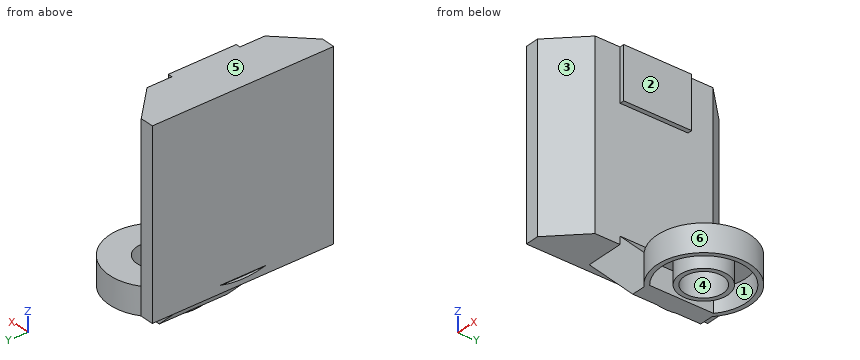
from build123d import *

# Parameters (mm, degrees)
F0_R     = 10.25
F0_R_2   = 4.25
F1_DEPTH = 6
F2_T     = -1
F4_DEPTH = 7.5
F6_DEPTH = 10
F7_SIZE  = 7


# Not quite as in the source:
# - a feature names something its author has since deleted; it is built from what else it names


with BuildPart() as f1:
    # F0 (on Top) → F1 (new body)
    with BuildSketch(Plane.XY):
        Circle(F0_R)
        Circle(F0_R_2, mode=Mode.SUBTRACT)
    extrude(amount=F1_DEPTH)

    # F2
    f2_openings = [f1.faces().sort_by_distance(p)[0] for p in [
        (-9.960086, 0, 0),
    ]]
    offset(amount=F2_T, openings=f2_openings)

    # F3 (on Front) → F4 (join, symmetric)
    with BuildSketch(Plane.XZ):
        Polygon((-23.44, 51.75), (-23.44, 13.44), (-10, 0), (-6, 0), (-6, 6), (-13.44, 13.44), (-13.44, 40.35), (-12.44, 40.35), (-12.44, 51.75), align=None)
    extrude(amount=F4_DEPTH, both=True)

    # F5 (on face) → F6 (join, through all)
    with BuildSketch(Plane(origin=(-23.44, 0, 0), x_dir=(0, -1, 0), z_dir=(-1, 0, 0))):
        with BuildLine():
            Line((20, 11.75), (20, 51.75))
            Line((20, 51.75), (7.5, 51.75))
            Line((7.5, 51.75), (7.5, 49.2070902501))
            ThreePointArc((7.5, 49.2070902501), (15.8666316526, 42.2022724802), (19, 31.75))
            ThreePointArc((19, 31.75), (15.8666316526, 21.2977275198), (7.5, 14.2929097499))
            Line((7.5, 14.2929097499), (7.5, 13.44))
            Line((7.5, 13.44), (5.0738446961, 13.44))
            ThreePointArc((5.0738446961, 13.44), (0, 12.75), (-5.0738446961, 13.44))
            Line((-5.0738446961, 13.44), (-7.5, 13.44))
            Line((-7.5, 13.44), (-7.5, 14.2929097499))
            ThreePointArc((-7.5, 14.2929097499), (-19, 31.75), (-7.5, 49.2070902501))
            Line((-7.5, 49.2070902501), (-7.5, 51.75))
            Line((-7.5, 51.75), (-20, 51.75))
            Line((-20, 51.75), (-20, 11.75))
            Line((-20, 11.75), (20, 11.75))
        make_face()
        with BuildLine():
            ThreePointArc((19, 31.75), (15.8666316526, 42.2022724802), (7.5, 49.2070902501))
            Line((7.5, 49.2070902501), (7.5, 14.2929097499))
            ThreePointArc((7.5, 14.2929097499), (15.8666316526, 21.2977275198), (19, 31.75))
        make_face()
        with BuildLine():
            Line((-7.5, 14.2929097499), (-7.5, 49.2070902501))
            ThreePointArc((-7.5, 49.2070902501), (-19, 31.75), (-7.5, 14.2929097499))
        make_face()
    extrude(amount=-F6_DEPTH)

    # F7
    f7_edges = [f1.edges().sort_by_distance(p)[0] for p in [
        (-13.44, -20, 31.75),
        (-13.44, 20, 31.75),
    ]]
    chamfer(f7_edges, length=F7_SIZE)


solid = f1.part
Source: CAD feature listing. Evaluate the final solid. Frame: model axes, mm. Face numbers are marked on the shaded views. A direction names the side the tool comes from. Round coordinates to 2 decimals unless told otherwise and drop trailing zeros. Loops run counter-clockwise (first coordinate to the right, second up) from the corner with the lowest first, then second, coordinate; pieces in that order, holes last. Notation, with made-up numbers: (1, 61.5) -> (59, 61.5) arc R29 ccw to (59, 99.5) -> close; hole circle Ø11 at (61.25, 35). An arc over 180 degrees is marked (long way). Answer as a JSON object with one key per item and string values. Group by question number.
Q1. Section query A-A (y = 0). Output: boundary loops of the cut face in (x, z).
Q2. Section query B-B (x = 0). Output: boundary loops of the cut face in (y, z), plus the area to 3 significant figures.
Q3. Access query for the marked faces 1, 2 and 3. Directions: +Z, -Z, +X, -X, +Y, -Y. A direction counts if a zero-diameter tool reaches every point of the face in a straight line with its end or side. Return the directions, or none.
Q4. Section query D-D (z = 27.5). Output: boundary loops of the cut face in (x, y), plus the area to 3 significant figures.
Q5. Section query C-C (x = -18). Output: boundary loops of the cut face in (y, z), plus the area to 3 significant figures.
Q6. Mould query, pull axis Y, two halves, no side actions, for the marked faces 4, 5 and 6. Classes: pulls with the +Y half, pulls with the -Y half, needs draft (parallel to the pull), parting line crosses it, or undercut.
Q7. Ray query, line 1 (Y direction, x = 0, z = 2.1); line 2 (X direction, y = -5, z = 14.5); line 3 (Z direction, x = -18, y = -15.5). Return the intervals inside material, ascending. Write a range as from..to.
Q8. Contact query for flat-ended pins moving along their axis: P1, Ø0.8, axis at x = -13, y = -2, coming from the -Z side; P2, Ø3, axis at y = -3, z = 36.5, coming from the +X side; P3, Ø2, axis at x = -7, y = -1.5, coming from the +Z side. Output: stop coordinate, or through.
Completed:
{
 "1": {"outline": "(-23.44, 11.75) -> (-21.75, 11.75) -> (-10.25, 0.25) -> (-10.25, 0) -> (-6, 0) -> (-6, 5) -> (-5.25, 5) -> (-5.25, 0) -> (-4.25, 0) -> (-4.25, 6) -> (-6, 6) -> (-13.44, 13.44) -> (-13.44, 40.35) -> (-12.44, 40.35) -> (-12.44, 51.75) -> (-23.44, 51.75) -> (-23.44, 13.44) -> (-22.75, 12.75) -> (-23.44, 12.75) -> close; (4.25, 0) -> (5.25, 0) -> (5.25, 5) -> (9.25, 5) -> (9.25, 0) -> (10.25, 0) -> (10.25, 6) -> (4.25, 6) -> close"},
 "2": {"outline": "(-10.25, 0) -> (-9.25, 0) -> (-9.25, 5) -> (-5.25, 5) -> (-5.25, 0) -> (-4.25, 0) -> (-4.25, 6) -> (-10.25, 6) -> close; (4.25, 0) -> (5.25, 0) -> (5.25, 5) -> (9.25, 5) -> (9.25, 0) -> (10.25, 0) -> (10.25, 6) -> (4.25, 6) -> close", "area": "32.0 mm²"},
 "3": {"face 1": "-Z", "face 2": "+Z, +X, +Y, -Y", "face 3": "+Z, -Z, +X, -Y"},
 "4": {"outline": "(-23.44, -20) -> (-20.44, -20) -> (-13.44, -13) -> (-13.44, 13) -> (-20.44, 20) -> (-23.44, 20) -> close", "area": "351 mm²"},
 "5": {"outline": "(-17.56, 11.75) -> (-7.5, 11.75) -> (-7.5, 8) -> (7.5, 8) -> (7.5, 11.75) -> (17.56, 11.75) -> (17.56, 51.75) -> (-17.56, 51.75) -> close", "area": "1,460 mm²"},
 "6": {"face 4": "undercut", "face 5": "needs draft", "face 6": "parting line crosses it"},
 "7": {"line 1": "-10.25..-9.25, -5.25..-4.25, 4.25..5.25, 9.25..10.25", "line 2": "-23.44..-13.44", "line 3": "11.75..51.75"},
 "8": {"P1": "z = 2.6", "P2": "x = -13.44", "P3": "z = 8"}
}
